from build123d import *

# Parameters (mm, degrees)
ESQUISSE1_W                = 48
ESQUISSE1_H                = 24
EXTRUSION1_DEPTH           = 7.5
CONG_2_R                   = 5
CONG_5_R                   = 1
CONG_6_R                   = 1
ESQUISSE4_W                = 0.5
ESQUISSE4_H                = 18.982849842
EXTRUSION2_DEPTH           = 0.5
ESQUISSE5_R                = 0.25
EXTRUSION3_DEPTH           = 0.5
CHANFREIN1_SIZE            = 1
ESQUISSE9_R                = 1.5
EXTRUSION6_DEPTH           = 0.5
EXTRUSION6_DRAFT           = -45
EXTRUSION6_PROFILE_2_DEPTH = 0.5
EXTRUSION6_PROFILE_2_DRAFT = -45
EXTRUSION6_PROFILE_3_DEPTH = 0.5
EXTRUSION6_PROFILE_3_DRAFT = -45
ESQUISSE10_R               = 2
EXTRUSION7_DEPTH           = 0.5
EXTRUSION7_DRAFT           = -45
EXTRUSION7_PROFILE_2_DEPTH = 0.5
EXTRUSION7_PROFILE_2_DRAFT = -45


with BuildPart() as part:
    # Esquisse1 → Extrusion1 (new body)
    with BuildSketch(Plane(origin=(0, 0, 0), x_dir=(1, 0, 0), z_dir=(0, 1, 0))):
        with Locations((24, 12)):
            Rectangle(ESQUISSE1_W, ESQUISSE1_H)
    extrude(amount=EXTRUSION1_DEPTH)

    # Congé2
    cong_2_edges = [part.edges().sort_by_distance(p)[0] for p in [
        (0, 3.75, -24),
        (48, 3.75, -24),
        (48, 3.75, 0),
        (0, 3.75, 0),
    ]]
    fillet(cong_2_edges, radius=CONG_2_R)

    # Congé5
    cong_5_edges = [part.edges().sort_by_distance(p)[0] for p in [
        (48, 7.5, -12),
        (24, 7.5, 0),
        (0, 7.5, -12),
        (24, 7.5, -24),
        (1.464466094, 7.5, -22.535533906),
        (1.464466094, 7.5, -1.464466094),
        (46.535533906, 7.5, -22.535533906),
        (46.535533906, 7.5, -1.464466094),
    ]]
    fillet(cong_5_edges, radius=CONG_5_R)

    # Congé6
    cong_6_edges = [part.edges().sort_by_distance(p)[0] for p in [
        (48, 0, -12),
        (0, 0, -12),
        (24, 0, -24),
        (24, 0, 0),
        (1.464466094, 0, -22.535533906),
        (1.464466094, 0, -1.464466094),
        (46.535533906, 0, -22.535533906),
        (46.535533906, 0, -1.464466094),
    ]]
    fillet(cong_6_edges, radius=CONG_6_R)

    # Esquisse4 → Extrusion2 (cut)
    with BuildSketch(Plane(origin=(0, 7.5, 0), x_dir=(1, 0, 0), z_dir=(0, 1, 0))):
        with Locations((24, 12)):
            Rectangle(ESQUISSE4_W, ESQUISSE4_H)
    extrude(amount=-EXTRUSION2_DEPTH, mode=Mode.SUBTRACT)

    # Esquisse5 → Extrusion3 (cut)
    with BuildSketch(Plane(origin=(0, 7.5, 0), x_dir=(1, 0, 0), z_dir=(0, 1, 0))):
        with Locations((24, 21.491424921)):
            Circle(ESQUISSE5_R)
        with Locations((24, 2.508575079)):
            Circle(ESQUISSE5_R)
    extrude(amount=-EXTRUSION3_DEPTH, mode=Mode.SUBTRACT)

    # Chanfrein1
    # the kernel refuses this chamfer: 1 mm, written as the material it takes off along each edge
    with BuildSketch(Plane(origin=(24, 7.5, -21.491424921), x_dir=(1, 0, 0), z_dir=(0, 0, 1))) as chanfrein1_piece_1_section:
        Polygon((0.25 + CHANFREIN1_SIZE, 0), (0.25, -CHANFREIN1_SIZE), (0.25, 0), align=None)
    chanfrein1_piece_1 = revolve(axis=Axis((24, 7.5, -21.491424921), (0, 1, 0)), revolution_arc=180, mode=Mode.PRIVATE)
    chanfrein1_piece_1 = split(chanfrein1_piece_1, bisect_by=Plane(origin=(24, 7, -21.964580549), z_dir=(0, 1, 0)), keep=Keep.TOP, mode=Mode.PRIVATE)
    add(chanfrein1_piece_1, mode=Mode.SUBTRACT)
    with BuildSketch(Plane(origin=(24.25, 7.5, -21.491424921), x_dir=(0.9996219169112968, 0.02749587661058651, 0), z_dir=(0, 0, 1))) as chanfrein1_piece_2_section:
        Polygon((CHANFREIN1_SIZE * 0.999621916911, -CHANFREIN1_SIZE * 0.0274958766106), (-CHANFREIN1_SIZE * 0.0274958766106, -CHANFREIN1_SIZE * 0.999621916911), (0, 0), align=None)
    chanfrein1_piece_2 = extrude(amount=18.982849842, mode=Mode.PRIVATE)
    chanfrein1_piece_2 = split(chanfrein1_piece_2, bisect_by=Plane(origin=(24.643401084, 7, -12), z_dir=(0, 1, 0)), keep=Keep.TOP, mode=Mode.PRIVATE)
    add(chanfrein1_piece_2, mode=Mode.SUBTRACT)
    with BuildSketch(Plane(origin=(24, 7.5, -2.508575079), x_dir=(-1, 0, 0), z_dir=(0, 0, -1))) as chanfrein1_piece_3_section:
        Polygon((0.25 + CHANFREIN1_SIZE, 0), (0.25, -CHANFREIN1_SIZE), (0.25, 0), align=None)
    chanfrein1_piece_3 = revolve(axis=Axis((24, 7.5, -2.508575079), (0, 1, 0)), revolution_arc=180, mode=Mode.PRIVATE)
    chanfrein1_piece_3 = split(chanfrein1_piece_3, bisect_by=Plane(origin=(24, 7, -2.035419451), z_dir=(0, 1, 0)), keep=Keep.TOP, mode=Mode.PRIVATE)
    add(chanfrein1_piece_3, mode=Mode.SUBTRACT)
    with BuildSketch(Plane(origin=(23.75, 7.5, -2.508575079), x_dir=(-0.9996219169112968, 0.02749587661058651, 0), z_dir=(0, 0, -1))) as chanfrein1_piece_4_section:
        Polygon((CHANFREIN1_SIZE * 0.999621916911, -CHANFREIN1_SIZE * 0.0274958766106), (-CHANFREIN1_SIZE * 0.0274958766106, -CHANFREIN1_SIZE * 0.999621916911), (0, 0), align=None)
    chanfrein1_piece_4 = extrude(amount=18.982849842, mode=Mode.PRIVATE)
    chanfrein1_piece_4 = split(chanfrein1_piece_4, bisect_by=Plane(origin=(23.356598916, 7, -12), z_dir=(0, 1, 0)), keep=Keep.TOP, mode=Mode.PRIVATE)
    add(chanfrein1_piece_4, mode=Mode.SUBTRACT)


with BuildPart() as extrusion6_tool:
    # Esquisse9 → Extrusion6 (with draft: the straight prism first)
    with BuildSketch(Plane(origin=(0, 7.5, 0), x_dir=(1, 0, 0), z_dir=(0, 1, 0))):
        with Locations((30.25, 18)):
            Circle(ESQUISSE9_R)
    extrude(amount=-EXTRUSION6_DEPTH)
    # Extrusion6: the draft: its side faces are tilted about the plane it starts from
    extrusion6_sides = [extrusion6_tool.faces().sort_by_distance(p)[0] for p in [
        (28.75, 7.25, -18),
    ]]
    draft(extrusion6_sides, Plane(origin=(0, 7.5, 0), x_dir=(1, 0, 0), z_dir=(0, 1, 0)), EXTRUSION6_DRAFT)


with BuildPart() as part_1:
    add(part.part)

    # Extrusion6: cut by extrusion6_tool
    add(extrusion6_tool.part, mode=Mode.SUBTRACT)


with BuildPart() as extrusion6_profile_2_tool:
    # Esquisse9 → Extrusion6 profile 2 (with draft: the straight prism first)
    with BuildSketch(Plane(origin=(0, 7.5, 0), x_dir=(1, 0, 0), z_dir=(0, 1, 0))):
        with Locations((36.125, 12)):
            Circle(ESQUISSE9_R)
    extrude(amount=-EXTRUSION6_PROFILE_2_DEPTH)
    # Extrusion6 profile 2: the draft: its side faces are tilted about the plane it starts from
    extrusion6_profile_2_sides = [extrusion6_profile_2_tool.faces().sort_by_distance(p)[0] for p in [
        (34.625, 7.25, -12),
    ]]
    draft(extrusion6_profile_2_sides, Plane(origin=(0, 7.5, 0), x_dir=(1, 0, 0), z_dir=(0, 1, 0)), EXTRUSION6_PROFILE_2_DRAFT)


with BuildPart() as part_2:
    add(part_1.part)

    # Extrusion6 profile 2: cut by extrusion6_profile_2_tool
    add(extrusion6_profile_2_tool.part, mode=Mode.SUBTRACT)


with BuildPart() as extrusion6_profile_3_tool:
    # Esquisse9 → Extrusion6 profile 3 (with draft: the straight prism first)
    with BuildSketch(Plane(origin=(0, 7.5, 0), x_dir=(1, 0, 0), z_dir=(0, 1, 0))):
        with Locations((42, 6)):
            Circle(ESQUISSE9_R)
    extrude(amount=-EXTRUSION6_PROFILE_3_DEPTH)
    # Extrusion6 profile 3: the draft: its side faces are tilted about the plane it starts from
    extrusion6_profile_3_sides = [extrusion6_profile_3_tool.faces().sort_by_distance(p)[0] for p in [
        (40.5, 7.25, -6),
    ]]
    draft(extrusion6_profile_3_sides, Plane(origin=(0, 7.5, 0), x_dir=(1, 0, 0), z_dir=(0, 1, 0)), EXTRUSION6_PROFILE_3_DRAFT)


with BuildPart() as part_3:
    add(part_2.part)

    # Extrusion6 profile 3: cut by extrusion6_profile_3_tool
    add(extrusion6_profile_3_tool.part, mode=Mode.SUBTRACT)


with BuildPart() as extrusion7_tool:
    # Esquisse10 → Extrusion7 (with draft: the straight prism first)
    with BuildSketch(Plane(origin=(0, 7.5, 0), x_dir=(1, 0, 0), z_dir=(0, 1, 0))):
        with Locations((7, 17)):
            Circle(ESQUISSE10_R)
    extrude(amount=-EXTRUSION7_DEPTH)
    # Extrusion7: the draft: its side faces are tilted about the plane it starts from
    extrusion7_sides = [extrusion7_tool.faces().sort_by_distance(p)[0] for p in [
        (5, 7.25, -17),
    ]]
    draft(extrusion7_sides, Plane(origin=(0, 7.5, 0), x_dir=(1, 0, 0), z_dir=(0, 1, 0)), EXTRUSION7_DRAFT)


with BuildPart() as part_4:
    add(part_3.part)

    # Extrusion7: cut by extrusion7_tool
    add(extrusion7_tool.part, mode=Mode.SUBTRACT)


with BuildPart() as extrusion7_profile_2_tool:
    # Esquisse10 → Extrusion7 profile 2 (with draft: the straight prism first)
    with BuildSketch(Plane(origin=(0, 7.5, 0), x_dir=(1, 0, 0), z_dir=(0, 1, 0))):
        with Locations((16.75, 7)):
            Circle(ESQUISSE10_R)
    extrude(amount=-EXTRUSION7_PROFILE_2_DEPTH)
    # Extrusion7 profile 2: the draft: its side faces are tilted about the plane it starts from
    extrusion7_profile_2_sides = [extrusion7_profile_2_tool.faces().sort_by_distance(p)[0] for p in [
        (14.75, 7.25, -7),
    ]]
    draft(extrusion7_profile_2_sides, Plane(origin=(0, 7.5, 0), x_dir=(1, 0, 0), z_dir=(0, 1, 0)), EXTRUSION7_PROFILE_2_DRAFT)


with BuildPart() as part_5:
    add(part_4.part)

    # Extrusion7 profile 2: cut by extrusion7_profile_2_tool
    add(extrusion7_profile_2_tool.part, mode=Mode.SUBTRACT)


solid = part_5.part
The model under review builds one solid part; all positions refer to its coordinate system, in mm. A direction names the side the tool comes from. Round coordinates to 2 decimals unless told otherwise and drop trailing zeros. Order: outer loops, then holes, each group sorted by start corner. A loop starts at its lowest first (then second) coordinate and runs counter-clockwise, first axis right, second up. Notation, with made-up numbers: (-29, -22) - (-3, -22) arc R20 cw to (-3, -2) - close; hole circle Ø1 at (-3.75, -26). An arc over 180 degrees is marked (long way). Use one line per item in the form item = value.
Q1. Tool access review of faces 5 (the cylindrical face through (0.301, 0.285, -11.902)), 6 (the flat face through (30, 7, -18)): name each direction out of +Z, -Z, +X, -X, +Y, -Y from which nothing blocks a thin tool from reaching the whole face with its end or side.
Response values:
face_5 = +Z, -Z, -X, -Y
face_6 = +Y
Q2. To check wall thickness, follow line 1 (X direction, y = 0.5, z = -10.5); line 2 (Z direction, x = 33.5, y = 7); line 3 (Z direction, x = 45.5, y = 3.5). State the ranges of each line that lie inside material, in increasing order.
Response values:
line_1 = 0.13 to 47.87
line_2 = -23.87 to -0.13
line_3 = -23.33 to -0.67
Q3. Clearance check with flat-ended pins moving along their axes: P1, Ø1.6, axis at x = 30.5, z = -18, coming from the +Y side; P2, Ø0.6, axis at x = 36.5, z = -12, coming from the +Y side; P3, Ø1.6, axis at x = 42, z = -5.5, coming from the +Y side. State where each tip first meets the part, or that it passes through.
Response values:
P1 = 7.05
P2 = 7
P3 = 7.3
Q4. Mouldability with a two-part tool opening along Z and no side actions: class faces 1 (the flat face through (48, 4, -12)), 2 (the cylindrical face through (23.734, 7.215, -23.699)), 3 (the flat face through (7, 7, -17)), 4 (the conical face through (23.98, 7.14, -1.62)) as pulls with the +Z half, pulls with the -Z half, needs draft (parallel to the pull), parting line crosses it, or undercut.
Response values:
face_1 = needs draft
face_2 = pulls with the -Z half
face_3 = undercut
face_4 = undercut
Q5. Add section B-B on x = 24. Give the boundary of the cut face in (y, z).
Response values:
outline = (0, -23) arc R1 ccw to (1, -24) - (6.5, -24) arc R1 ccw to (7.5, -23) - (7.5, -22.74) - (7, -22.24) - (7, -1.76) - (7.5, -1.26) - (7.5, -1) arc R1 ccw to (6.5, 0) - (1, 0) arc R1 ccw to (0, -1) - close
Q6. Add section A-A on y = 2. Give the boundary of the cut face in (x, z), then the cut area to 3 significant figures.
Response values:
outline = (0, -19) arc R5 ccw to (5, -24) - (43, -24) arc R5 ccw to (48, -19) - (48, -5) arc R5 ccw to (43, 0) - (5, 0) arc R5 ccw to (0, -5) - close
area = 1,130 mm^2
